Autodesk Inventor part; units mm, degrees
ref_plane "YZ Plane" through (0, 0, 0) normal (1, 0, 0) x (0, 1, 0)
ref_plane "XZ Plane" through (0, 0, 0) normal (0, 1, 0) x (-1, 0, 0)
ref_plane "XY Plane" through (0, 0, 0) normal (0, 0, 1) x (1, 0, 0)
sketch "Esquisse1" plane through (0, 0, 0) normal (0, 1, 0) x (-1, 0, 0)
  circle A0 centre (0, 0) radius 31.5
  dimension "d0" = 63
extrude "Extrusion1" add sketch "Esquisse1" along normal blind 127
sketch "Esquisse2" plane through (0, 127, 0) normal (0, 1, 0) x (1, 0, 0)
  circle A0 centre (0, 0) radius 31.5
  circle A1 centre (0, 0) radius 12.5
  dimension "d3" = 25
extrude "Extrusion2" add sketch "Esquisse2" along normal blind 2.5 contours A1
sketch "Esquisse3" plane through (0, 0, 0) normal (0, -1, 0) x (1, 0, 0)
  circle A0 centre (0, 0) radius 31.5
  circle A1 centre (0, 0) radius 12.5
  dimension "d6" = 25
extrude "Extrusion3" add sketch "Esquisse3" along normal blind 3.7 contours A1
sketch "Esquisse4" plane through (0, -3.7, 0) normal (0, -1, 0) x (1, 0, 0)
  circle A0 centre (0, 0) radius 12.5
  circle A1 centre (0, 0) radius 4
  dimension "d9" = 8
extrude "Extrusion4" add sketch "Esquisse4" along normal blind 21.3 contours A1
chamfer "Chanfrein1" distance 0.5 angle 45 1 edges at (-4, -25, 0)
sketch "Esquisse5" plane through (0, 0, 0) normal (0, -1, 0) x (1, 0, 0)
  circle A0 centre (0, 0) radius 12.5
  circle A1 centre (0, 20) radius 2.5
  dimension "d15" = 5
  dimension "d16" = 20
extrude "Extrusion5" cut sketch "Esquisse5" against normal blind 10 contours A1
pattern_circular "Réseau circulaire1" count 4 over 360 about axis through (0, -3.7, 0) along (0, -1, 0) of "Extrusion5"
sketch "Esquisse6" plane through (0, 127, 0) normal (0, 1, 0) x (1, 0, 0)
  circle A0 centre (0, 0) radius 12.5
  circle A1 centre (0, 20) radius 2.5
  dimension "d22" = 5
  dimension "d23" = 20
extrude "Extrusion6" cut sketch "Esquisse6" against normal blind 7 contours A1
pattern_circular "Réseau circulaire2" count 4 over 360 about axis through (0, 127, 0) along (0, 1, 0) of "Extrusion6"
properties part number "Moteur Crouzet" material "Acier inoxydable"
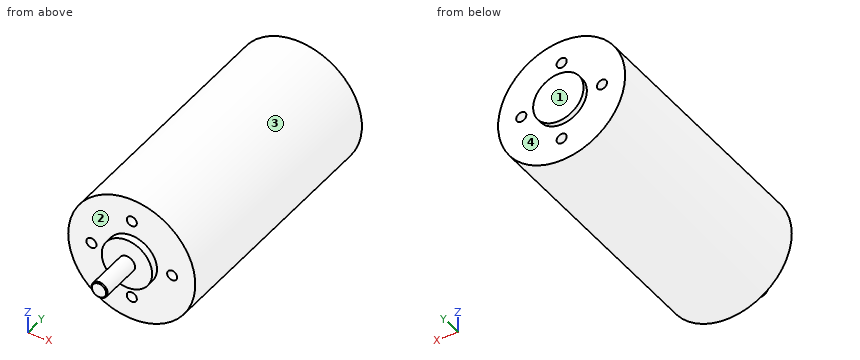
Model file for the job. Use its own axes, mm. Face numbers are marked on the shaded views. A direction names the side the tool comes from. Coordinates: 2 decimals unless noted, no trailing zeros. Write each loop counter-clockwise with the first axis right and the second up, starting at its lowest first coordinate (ties: lowest second). Pieces come first, ordered by that corner, then holes. Notation, with made-up numbers: (34.25, 17.25) -> (72.25, 17.25) arc R21 cw to (72.25, 42.25) -> close; hole circle Ø5 at (58.5, 9.5). An arc over 180 degrees is marked (long way). One line per item, written item: value. Start each with the question number.
1) Which spindle directions (+Z, -Z, +X, -X, +Y, -Y) get a long thin tool onto all of the face, cutting with end or side? Do the marked faces 1 and 2. Say none if no direction does.
2) Slice it at B-B on y = -8.5. Write the cut outline in (x, z), then the cut area to 3 significant figures.
3) Flat gauge pins, fed straight in: pin 1 Ø6 at (y, z) = (75, 21) entering from -X; pin 2 Ø1.5 at (x, z) = (20.5, -1) entering from +Y; pin 3 Ø3 at (x, y) = (-4.5, 36) entering from -Z. Where does each tip first touch, or does it go through?
4) Slice it at D-D on x = -10.5. Write the cut outline in (y, z).
5) Slice it at C-C on x = -20. Write the cut outline in (y, z).
6) Pull direction Z, two halves, no side cores. Call the marked faces 3 and 4: +Z half, -Z half, draft (parallel to the pull), parting line (faces both ways), or undercut.
7) Probe probe 1 along Z at (x, y) = (0, 125.5); probe 2 along Y at (x, z) = (12, -18); probe 3 along Y at (x, z) = (-1.5, 19). List the from-to ranges inside material, lowest first.
Answers follow:
1. face 1: +Z, -Z, +X, -X, +Y
1. face 2: -Y
2. outline: circle Ø8 at (0, 0)
2. area: 50.3 mm2
3. pin 1: x = -25.85
3. pin 2: y = 120
3. pin 3: z = -31.36
4. outline: (-3.7, -6.78) -> (0, -6.78) -> (0, -29.7) -> (127, -29.7) -> (127, -6.78) -> (129.5, -6.78) -> (129.5, 6.78) -> (127, 6.78) -> (127, 29.7) -> (0, 29.7) -> (0, 6.78) -> (-3.7, 6.78) -> close
5. outline: (0, -24.34) -> (127, -24.34) -> (127, -2.5) -> (120, -2.5) -> (120, 2.5) -> (127, 2.5) -> (127, 24.34) -> (0, 24.34) -> (0, 2.5) -> (10, 2.5) -> (10, -2.5) -> (0, -2.5) -> close
6. face 3: parting line
6. face 4: draft
7. probe 1: -31.5 to -22.5, -17.5 to 17.5, 22.5 to 31.5
7. probe 2: 0 to 127
7. probe 3: 10 to 120
